Autodesk Inventor part; units mm, degrees
ref_plane "YZ Plane" through (0, 0, 0) normal (1, 0, 0) x (0, 1, 0)
ref_plane "XZ Plane" through (0, 0, 0) normal (0, 1, 0) x (-1, 0, 0)
ref_plane "XY Plane" through (0, 0, 0) normal (0, 0, 1) x (1, 0, 0)
sketch "Sketch1" plane through (0, 0, 0) normal (0, 1, 0) x (-1, 0, 0)
  circle A0 centre (0, 0) radius 2.44
  circle A1 centre (0, 0) radius 4.2
  line L0 (1.1547, -2) -> (-1.1547, -2)
  line L1 (-1.1547, -2) -> (-2.3094, 0)
  line L2 (-2.3094, 0) -> (-1.1547, 2)
  line L3 (-1.1547, 2) -> (1.1547, 2)
  line L4 (1.1547, 2) -> (2.3094, 0)
  line L5 (2.3094, 0) -> (1.1547, -2)
  dimension "d0" = 4.88
  dimension "d1" = 8.4
  dimension "d8" = 4
extrude "Extrusion1" add sketch "Sketch1" along normal blind 5 contours A0 | A1 | L0 L1 L2 L3 L4 L5
extrude "Extrusion2" add sketch "Sketch1" against normal blind 12 contours A0 | L0 L1 L2 L3 L4 L5
extrude "Extrusion3" cut sketch "Sketch1" against normal blind 3 from surface at 5 contours L0 L1 L2 L3 L4 L5
fillet "Fillet1" radius 0.5 1 edges at (4.2, 5, 0)
thread "Thread2"
equation "\"d4\" = length"
equation "\"length\" = 12"
properties part number "M5x12"
Part model, mm, in its own coordinate system. A direction names the side the tool comes from. Round coordinates to 2 decimals unless told otherwise and drop trailing zeros. Write each loop counter-clockwise with the first axis right and the second up, starting at its lowest first coordinate (ties: lowest second). Pieces come first, ordered by that corner, then holes. Notation, with made-up numbers: (37.25, -13) - (67.25, -13) arc R15 cw to (67.25, -7) - close; hole circle Ø11 at (17.25, 8). An arc over 180 degrees is marked (long way). Use CSV: the item, a comma, the result in double quotes.
Item 1: Wall check: L1, parallel to Y at x = 3, z = 1; L2, parallel to X at y = 3, z = 1.5; L3, parallel to Y at x = 1, z = 1.5. Give the ranges that are in metal, low to high.
Results list:
L1,"y = 0 to 5"
L2,"x = -3.92 to -1.44, 1.44 to 3.92"
L3,"y = -12 to 2"
Item 2: Pull direction Z, two halves, no side cores. Call faces 1 (the flat face through (-2, 5, -2)), 2 (the cylindrical face through (-4.006, 2.218, -1.262)), 3 (the flat face through (0, 4, -2)): pulls with the +Z half, pulls with the -Z half, needs draft (parallel to the pull), parting line crosses it, or undercut.
Results list:
face 1,"needs draft"
face 2,"parting line crosses it"
face 3,"undercut"
Item 3: Slice it at A-A, the plane y = 2.75. Write the cut outline in (x, z), then the cut area to 3 significant figures.
Results list:
outline,"circle Ø8.4 at (0, 0); hole (-2.31, 0) - (-1.15, -2) - (1.15, -2) - (2.31, 0) - (1.15, 2) - (-1.15, 2) - close"
area,"41.6 mm²"
Item 4: Slice it at B-B, the plane x = 0. Write the cut outline in (y, z).
Results list:
outline,"(-12, -2.44) - (0, -2.44) - (0, -4.2) - (4.5, -4.2) arc R0.5 ccw to (5, -3.7) - (5, -2) - (2, -2) - (2, 2) - (5, 2) - (5, 3.7) arc R0.5 ccw to (4.5, 4.2) - (0, 4.2) - (0, 2.44) - (-12, 2.44) - close"
Item 5: Tool access for faces 4 (the flat face through (0, -12, 0)), 5 (the cylindrical face through (0.53, -5.92, -2.38)), 6 (the flat face through (-1.724, 3.521, 1.014)): list every direction of +Z, -Z, +X, -X, +Y, -Y with a clear straight run to the whole face (end or side of a thin tool).
Results list:
face 4,"+Z, -Z, +X, -X, -Y"
face 5,"-Y"
face 6,"+Y"
Item 6: Flat gauge pins, fed straight in: P1, Ø1.2, axis at x = -1, z = -1, coming from the +Y side; P2, Ø4, axis at x = -1.5, y = -4, coming from the -Z side; P3, Ø1, axis at x = -3, z = 2, coming from the -Y side. Where does each tip first touch, or does it go through?
Results list:
P1,"stops at y = 2"
P2,"stops at z = -2.44"
P3,"stops at y = 0"
Item 7: Slice it at C-C, the plane y = -2. Write the cut outline in (x, z), then the cut area to 3 significant figures.
Results list:
outline,"circle Ø4.88 at (0, 0)"
area,"18.7 mm²"
